Design review of the part built by this model. Coordinates are the model's own, in mm. Face numbers are marked on the shaded views. A direction names the side the tool comes from. Give positions to 0.01 mm unless a question says otherwise; leave off trailing zeros. Order: outer loops, then holes, each group sorted by start corner. A loop starts at its lowest first (then second) coordinate and runs counter-clockwise, first axis right, second up.
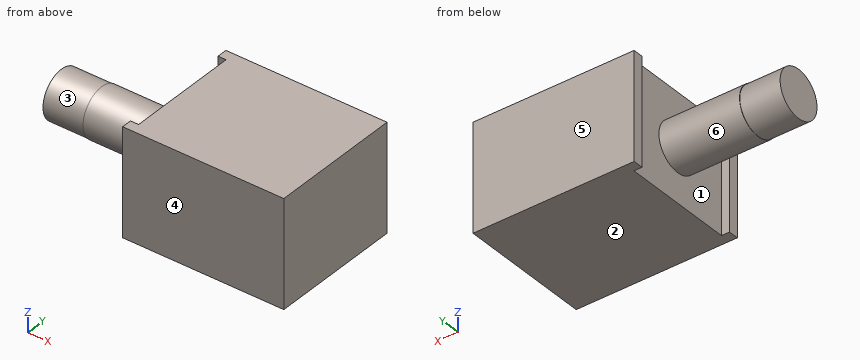
```python
from build123d import *

# Parameters (mm, degrees)
F0_W          = 20
F0_H          = 16.5
F1_DEPTH      = 6.65
F3_W          = 1
F3_H          = 14
F4_DEPTH      = 13.301
F2_R          = 3
F5_DEPTH      = 9
F5_DEPTH_BACK = 1
F6_R          = 2.95
F7_DEPTH      = 5


with BuildPart() as f1:
    # F0 (on Top) → F1 (new body, symmetric)
    with BuildSketch(Plane.XY):
        Rectangle(F0_W, F0_H)
    extrude(amount=F1_DEPTH, both=True)

    # F3 (on face) → F4 (cut, through all)
    with BuildSketch(Plane.XY.offset(6.65)):
        with Locations((-9.5, 0)):
            Rectangle(F3_W, F3_H)
    extrude(amount=-F4_DEPTH, mode=Mode.SUBTRACT)

    # F2 (on face) → F5 (join, two sides)
    with BuildSketch(Plane(origin=(-10, 0, 0), x_dir=(0, -1, 0), z_dir=(-1, 0, 0))) as f5_sk:
        Circle(F2_R)
    extrude(amount=F5_DEPTH)
    extrude(f5_sk.sketch, amount=-F5_DEPTH_BACK)

    # F6 (on face) → F7 (join)
    with BuildSketch(Plane(origin=(-19, 0, 0), x_dir=(0, -1, 0), z_dir=(-1, 0, 0))):
        Circle(F6_R)
    extrude(amount=F7_DEPTH)


solid = f1.part
```
1. For line 1 along X through (y, z) = (0.75, 3); line 2 along Y through (x, z) = (-22, -2.5); line 3 along Z through (x, y) = (-16.5, -1.5), list the stretches that pass through material, from the lowest coordinate up.
Recorded:
line 1: x = -9 to 10
line 2: y = -1.57 to 1.57
line 3: z = -2.6 to 2.6
2. Take a section at B-B (y = 0). State the section outline as (x, z) points, then the cut area to 3 significant figures.
Recorded:
outline: (-24, -2.95) - (-19, -2.95) - (-19, -3) - (-9, -3) - (-9, -6.65) - (10, -6.65) - (10, 6.65) - (-9, 6.65) - (-9, 3) - (-19, 3) - (-19, 2.95) - (-24, 2.95) - close
area: 342 mm2
3. Machinability: for the marked faces 5 and 6, which of the approach directions +Z, -Z, +X, -X, +Y, -Y give a long, thin tool a straight path to every point of the face, cutting with its end or side? Answer none if there is none.
Recorded:
face 5: +Z, -Z, +X, -X, +Y
face 6: -X
4. Draft analysis for pull direction Y (two halves, no side actions). For the marked faces 1, 2, 3 and 4, state which applies: pulls with the +Y half, pulls with the -Y half, needs draft (parallel to the pull), parting line crosses it, or undercut.
Recorded:
face 1: undercut
face 2: needs draft
face 3: parting line crosses it
face 4: pulls with the -Y half
5. Take a section at D-D (y = -6). State the section outline as (x, z) points.
Recorded:
outline: (-9, -6.65) - (10, -6.65) - (10, 6.65) - (-9, 6.65) - close
6. For pin 1 (8 mm diameter, centred on x = -15, y = -6, fed in from -Z); pin 2 (0.6 mm diameter, centred on y = -7.5, z = -3, fed in from -X); pin 3 (2 mm diameter, centred on x = -13.5, y = 0, fed in from +Z), all flat-tipped, find the tip position at first contact; note any pin that passes through.
Recorded:
pin 1: stops at z = -2.24
pin 2: stops at x = -10
pin 3: stops at z = 3
7. Take a section at C-C (z = 0). State the section outline as (x, y) points.
Recorded:
outline: (-24, -2.95) - (-19, -2.95) - (-19, -3) - (-9, -3) - (-9, -7) - (-10, -7) - (-10, -8.25) - (10, -8.25) - (10, 8.25) - (-10, 8.25) - (-10, 7) - (-9, 7) - (-9, 3) - (-19, 3) - (-19, 2.95) - (-24, 2.95) - close
8. Take a section at A-A (z = -3.75). State the section outline as (x, y) points, then the cut area to 3 significant figures.
Recorded:
outline: (-10, -8.25) - (10, -8.25) - (10, 8.25) - (-10, 8.25) - (-10, 7) - (-9, 7) - (-9, -7) - (-10, -7) - close
area: 316 mm2
